Geometry: see drawing. Coordinates: mm, zero at the bounding-box minimum. A direction names the side the tool comes from. Coordinates: 2 decimals unless noted, no trailing zeros. Loops run counter-clockwise (first coordinate to the right, second up) from the corner with the lowest first, then second, coordinate; pieces in that order, holes last. Notation, with made-up numbers: (-40, 43) - (10, 43) arc R20 cw to (10, 50) - close; hole circle Ø5 at (16.25, 63.5). An arc over 180 degrees is marked (long way). Use one line per item in the form item = value.
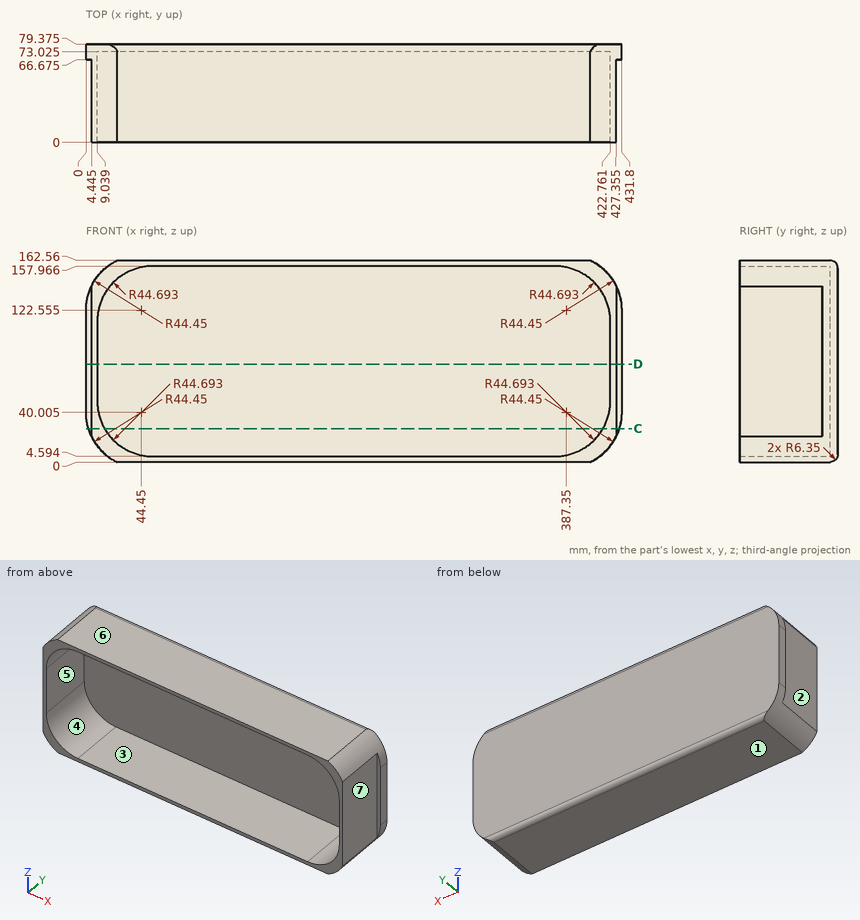
Q1. Cut plane C-C, the plane z = 27. Return loops of the section in (x, y) (1 decimal), then the cut area to 3 significant figures.
Check values:
outline = (1.9, 66.7) - (4.4, 66.7) - (4.4, 0) - (15, 0) - (15, 73) - (416.8, 73) - (416.8, 0) - (427.4, 0) - (427.4, 66.7) - (429.9, 66.7) - (429.9, 79.4) - (1.9, 79.4) - close
area = 4,290 mm²
Q2. Pull-direction query (X, two-part tool) for the marked faces 1, 2, 3 and 4; classes: pulls with the +X half, pulls with the -X half, needs draft (parallel to the pull), parting line crosses it, or undercut.
Check values:
face_1 = needs draft
face_2 = pulls with the -X half
face_3 = undercut
face_4 = undercut
Q3. Cut plane D-D, the plane z = 79. Return loops of the section in (x, y) (1 decimal), then the cut area to 3 significant figures.
Check values:
outline = (0, 66.7) - (4.4, 66.7) - (4.4, 0) - (9, 0) - (9, 73) - (422.8, 73) - (422.8, 0) - (427.4, 0) - (427.4, 66.7) - (431.8, 66.7) - (431.8, 79.4) - (0, 79.4) - close
area = 3,470 mm²
Q4. Ray query, line 1 along Z through (x, y) = (69.5, 47); line 2 along X through (y, z) = (29.5, 87) (1 decimal); line 3 along Y through (x, z) = (106, 33.5) (1 decimal). Return the intervals inside material, ascending. Write a range as [from, to].
Check values:
line_1 = [0, 4.59], [157.97, 162.56]
line_2 = [4.4, 9], [422.8, 427.4]
line_3 = [73, 79.4]
Q5. First-contact query: P1, Ø1.5, axis at y = 33.5, z = 50, coming from the -X side (3 decimals); P2, Ø5, axis at x = 64.5, z = 137.5, coming from the -Y side (3 decimals); P3, Ø8, axis at y = 56.5, z = 91.5, coming from the +X side (3 decimals). Flat tips, straight axial feed; report the tip coordinate or a pass-through.
Check values:
P1 = 4.445
P2 = 73.025
P3 = 427.355
Q6. Set-up query: the marked faces 5, 6 and 7. Return all of +Z, -Z, +X, -X, +Y, -Y with unobstructed straight access to the full face (end or side cutting, diameter ignored); none if empty.
Check values:
face_5 = -Y
face_6 = +Z, +X, -X, +Y, -Y
face_7 = +Z, -Z, +X, -Y
